Geometry: see drawing. Coordinates: mm, zero at the bounding-box minimum. Round coordinates to 2 decimals unless told otherwise and drop trailing zeros. Order: outer loops, then holes, each group sorted by start corner. A loop starts at its lowest first (then second) coordinate and runs counter-clockwise, first axis right, second up.
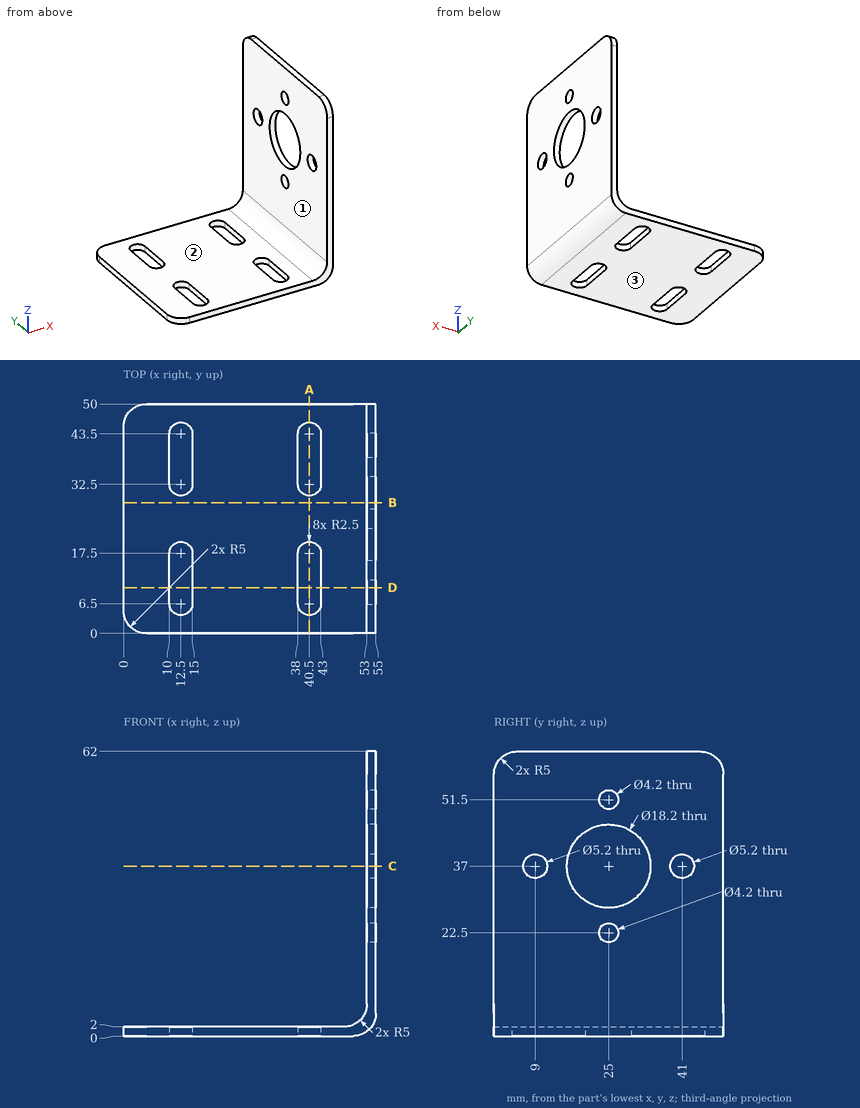
1. First-contact query: pin 1 (7 mm diameter, centred on y = 41, z = 37, fed in from -X); pin 2 (2 mm diameter, centred on y = 38, z = 1, fed in from +X); pin 3 (11 mm diameter, centred on y = 25, z = 37, fed in from +X); pin 4 (10 mm diameter, centred on x = 38, y = 26, fed in from +Z). Flat tips, straight axial feed; report the tip coordinate or a pass-through.
2. Line query: line 1 along Z through (x, y) = (54, 25); line 2 along Z through (x, y) = (54.45, 25); line 3 along Z through (x, y) = (24.5, 43). Output: solid intervals per line, ascending.
3. Section B-B on y = 28.5. Return loops of the section in (x, z).
4. Section C-C on z = 37. Return loops of the section in (x, y).
5. Section D-D on y = 10. Return loops of the section in (x, z).
6. Pull-direction query (Z, two-part tool) for the marked faces 1, 2 and 3; classes: released by +Z, released by -Z, zero draft, split by the parting line, or undercut.
7. Section A-A on x = 40.5. Return loops of the section in (y, z).
Result:
1. pin 1: stops at x = 53
1. pin 2: stops at x = 54
1. pin 3: passes through
1. pin 4: stops at z = 2
2. line 1: z = 2 to 20.4, 24.6 to 27.9, 46.1 to 49.4, 53.6 to 62
2. line 2: z = 2.72 to 20.4, 24.6 to 27.9, 46.1 to 49.4, 53.6 to 62
2. line 3: z = 0 to 2
3. outline: (0, 0) - (50, 0) arc R5 ccw to (55, 5) - (55, 28.6) - (53, 28.6) - (53, 7) arc R5 cw to (48, 2) - (0, 2) - close; (53, 45.4) - (55, 45.4) - (55, 62) - (53, 62) - close
4. outline: (53, 0) - (55, 0) - (55, 6.4) - (53, 6.4) - close; (53, 11.6) - (55, 11.6) - (55, 15.9) - (53, 15.9) - close; (53, 34.1) - (55, 34.1) - (55, 38.4) - (53, 38.4) - close; (53, 43.6) - (55, 43.6) - (55, 50) - (53, 50) - close
5. outline: (0, 0) - (10, 0) - (10, 2) - (0, 2) - close; (15, 0) - (38, 0) - (38, 2) - (15, 2) - close; (43, 0) - (50, 0) arc R5 ccw to (55, 5) - (55, 34.6) - (53, 34.6) - (53, 7) arc R5 cw to (48, 2) - (43, 2) - close; (53, 39.4) - (55, 39.4) - (55, 62) - (53, 62) - close
6. face 1: zero draft
6. face 2: released by +Z
6. face 3: released by -Z
7. outline: (0, 0) - (4, 0) - (4, 2) - (0, 2) - close; (20, 0) - (30, 0) - (30, 2) - (20, 2) - close; (46, 0) - (50, 0) - (50, 2) - (46, 2) - close
